```python
from build123d import *

# Parameters (mm, degrees)
F0_W      = 1219.2
F0_H      = 609.6
F0_W_2    = 1015.999996
F0_H_2    = 406.399996
F1_DEPTH  = 50.8
F2_W      = 1117.6
F2_H      = 508
F2_W_2    = 914.400004
F2_H_2    = 304.800004
F3_DEPTH  = 50.8
F4_W      = 1016
F4_H      = 406.4
F4_W_2    = 812.799998
F4_H_2    = 203.199998
F5_DEPTH  = 50.8
F6_W      = 914.4
F6_H      = 304.8
F6_W_2    = 711.199998
F6_H_2    = 101.599998
F7_DEPTH  = 50.8
F8_W      = 914.4
F8_H      = 304.8
F9_DEPTH  = 6.35
F10_W     = 50.8
F10_H     = 50.8
F11_DEPTH = 254
F13_W     = 914.4
F13_H     = 304.8
F14_DEPTH = 12.7


with BuildPart() as f1:
    # F0 (on Top) → F1 (new body)
    with BuildSketch(Plane.XY):
        Rectangle(F0_W, F0_H)
        Rectangle(F0_W_2, F0_H_2, mode=Mode.SUBTRACT)
    extrude(amount=F1_DEPTH)

    # F2 (on face) → F3 (join)
    with BuildSketch(Plane(origin=(0, 0, 0), x_dir=(1, 0, 0), z_dir=(0, 0, -1))):
        Rectangle(F2_W, F2_H)
        Rectangle(F2_W_2, F2_H_2, mode=Mode.SUBTRACT)
    extrude(amount=F3_DEPTH)

    # F4 (on face) → F5 (join)
    with BuildSketch(Plane(origin=(0, 0, -50.8), x_dir=(1, 0, 0), z_dir=(0, 0, -1))):
        Rectangle(F4_W, F4_H)
        Rectangle(F4_W_2, F4_H_2, mode=Mode.SUBTRACT)
    extrude(amount=F5_DEPTH)

    # F6 (on face) → F7 (join)
    with BuildSketch(Plane(origin=(0, 0, -101.6), x_dir=(1, 0, 0), z_dir=(0, 0, -1))):
        Rectangle(F6_W, F6_H)
        Rectangle(F6_W_2, F6_H_2, mode=Mode.SUBTRACT)
    extrude(amount=F7_DEPTH)

    # F8 (on face) → F9 (join)
    with BuildSketch(Plane(origin=(0, 0, -152.4), x_dir=(1, 0, 0), z_dir=(0, 0, -1))):
        Rectangle(F8_W, F8_H)
    extrude(amount=F9_DEPTH)

    # F10 (on face) → F11 (join)
    with BuildSketch(Plane(origin=(0, 0, -158.75), x_dir=(1, 0, 0), z_dir=(0, 0, -1))):
        with Locations((-431.8, 127)):
            Rectangle(F10_W, F10_H)
        with Locations((-431.8, -127)):
            Rectangle(F10_W, F10_H)
        with Locations((431.8, 127)):
            Rectangle(F10_W, F10_H)
        with Locations((431.8, -127)):
            Rectangle(F10_W, F10_H)
    extrude(amount=F11_DEPTH)

    # F13 (on offset) → F14 (join)
    with BuildSketch(Plane.XY.offset(-355.6)):
        Rectangle(F13_W, F13_H)
    extrude(amount=F14_DEPTH)


solid = f1.part
```
CAD build for the part. Positions are in the model's coordinates, mm. A direction names the side the tool comes from. Coordinates: 2 decimals unless noted, no trailing zeros. Order: outer loops, then holes, each group sorted by start corner. A loop starts at its lowest first (then second) coordinate and runs counter-clockwise, first axis right, second up. Notation, with made-up numbers: M 42,33.5 L 79,33.5 A17 cw 79,38.5 Z; hole C 51,31.5 d8. An arc over 180 degrees is marked long. Answer as CSV lines item,"result".
1) Cut at C-C (z = 17). List the corners of the cut face in (x, y).
Verdict:
outline,"M -609.6,-304.8 L 609.6,-304.8 L 609.6,304.8 L -609.6,304.8 Z; hole M -508,-203.2 L 508,-203.2 L 508,203.2 L -508,203.2 Z"
2) 3-axis set-ups, long thin cutter, end or side, ignore diameter. For faces 1 (the flat face through (-432, 101.6, -250)), 2 (the flat face through (-7, -203.2, -76)), 3 (the flat face through (-406.4, 1, -76)), 4 (the flat face through (558.8, 4, -25)): which of +Z, -Z, +X, -X, +Y, -Y reach the whole face in a straight line?
Verdict:
face 1,"+X, -X"
face 2,"-Z, +X, -X, -Y"
face 3,"+Z"
face 4,"-Z, +X, +Y, -Y"
3) Cut at D-D (y = 170.5). List the corners of the cut face in (x, z).
Verdict:
outline,"M -609.6,0 L -558.8,0 L -558.8,-50.8 L -508,-50.8 L -508,-101.6 L 508,-101.6 L 508,-50.8 L 558.8,-50.8 L 558.8,0 L 609.6,0 L 609.6,50.8 L 508,50.8 L 508,0 L -508,0 L -508,50.8 L -609.6,50.8 Z"
4) Cut at A-A (z = -243). List the corners of the cut face in (x, y), then the cut area to 3 significant figures.
Verdict:
outline,"M -457.2,-152.4 L -406.4,-152.4 L -406.4,-101.6 L -457.2,-101.6 Z; M -457.2,101.6 L -406.4,101.6 L -406.4,152.4 L -457.2,152.4 Z; M 406.4,-152.4 L 457.2,-152.4 L 457.2,-101.6 L 406.4,-101.6 Z; M 406.4,101.6 L 457.2,101.6 L 457.2,152.4 L 406.4,152.4 Z"
area,"10,300 mm2"
5) Flat gauge pins, fed straight in: P1, Ø1.5, axis at x = 53, z = -58.5, coming from the -Y side; P2, Ø1, axis at y = 55, z = -348.5, coming from the -X side; P3, Ø1, axis at x = -214, y = -121.5, coming from the +Z side. Where does each tip first touch, or does it go through?
Verdict:
P1,"y = -203.2"
P2,"x = -457.2"
P3,"z = -50.8"
6) Mould opens along Y. For faces 5 (the flat face through (-558.8, 4, -25)), 6 (the flat face through (-432, 101.6, -384)), 7 (the flat face through (-7, 203.2, -76)) say: released by +Y, released by -Y, zero draft, split by the parting line, or undercut.
Verdict:
face 5,"zero draft"
face 6,"undercut"
face 7,"released by +Y"
7) Drill centre lines: L1, parallel to Y at x = 128, z = -42.5; L2, parallel to Y at x = -417, z = -216.5; L3, parallel to X at y = -65, z = -69. Where is each one in solid material? Low to high. Write a range as from..to.
Verdict:
L1,"-254..-152.4, 152.4..254"
L2,"-152.4..-101.6, 101.6..152.4"
L3,"-508..-406.4, 406.4..508"
